Input: part model. Units: mm. Frame: model coordinates. Face numbers are marked on the shaded views. A direction names the side the tool comes from. Round coordinates to 2 decimals unless told otherwise and drop trailing zeros. Order: outer loops, then holes, each group sorted by start corner. A loop starts at its lowest first (then second) coordinate and runs counter-clockwise, first axis right, second up.
Item 1: First-contact query: pin 1 (3 mm diameter, centred on x = 9, y = -1, fed in from +Z); pin 2 (2 mm diameter, centred on y = -5, z = 5.5, fed in from +X); pin 3 (4.5 mm diameter, centred on x = 11, z = 3.5, fed in from -Y); pin 4 (1.6 mm diameter, centred on x = 10, y = -6, fed in from -Z). Flat tips, straight axial feed; report the tip coordinate or a pass-through.
Item 2: Mould query, pull axis Y, two halves, no side actions, for the marked faces 5, 6, 7 and 8. Classes: released by +Y, released by -Y, zero draft, split by the parting line, or undercut.
Item 3: Cut plane B-B on y = 7. Output: boundary loops of the cut face in (x, z).
Item 4: Line query: L1, parallel to Z at x = 4.75, y = -7.5; L2, parallel to Y at x = 5, z = 6 (3 decimals); L3, parallel to Y at x = -7.5, z = 3.6. Output: solid intervals per line, ascending.
Item 5: Cut plane C-C on x = 7.25. Output: boundary loops of the cut face in (y, z), then the cut area to 3 significant figures.
Item 6: Reachability of the marked faces 1, 2, 3 and 4 from +Z, -Z, +X, -X, +Y, -Y: full face, straight path, thin tool, end or side. Return the list, or none.
Item 7: Cut plane D-D on z = 2.75. Give the number of separate pieces and of enclosed holes in the cut face, then the cut area to 3 significant figures.
Item 8: Cut plane A-A on x = -9. Output: boundary loops of the cut face in (y, z).
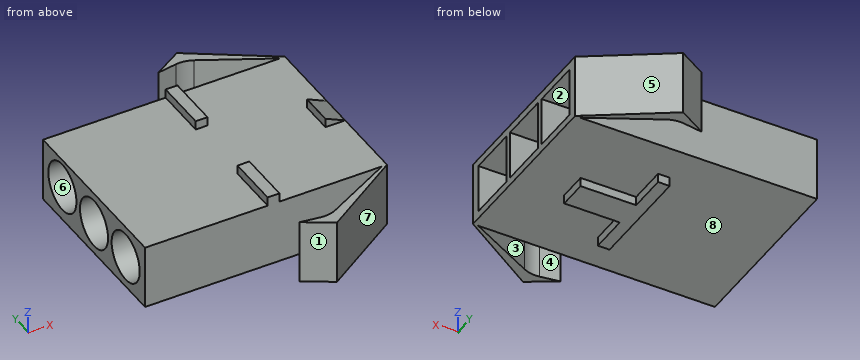
```python
from build123d import *

# Parameters (mm, degrees)
SKETCH_1_W          = 27
SKETCH_1_H          = 20
EXTRUDE_1_DEPTH     = 7.2
SKETCH_2_W          = 5.5
SKETCH_2_H          = 5.5
CUT_EXTRUDE_1_DEPTH = 10.2
SKETCH_3_R          = 2.75
CUT_EXTRUDE_2_DEPTH = 18
SKETCH_4_W          = 1.32
SKETCH_4_H          = 5.9
SKETCH_4_W_2        = 2.2
SKETCH_4_H_2        = 3.6
EXTRUDE_2_DEPTH     = 1
CHAMFER_1_SIZE      = 1
CHAMFER_1_SIZE2     = 2.144506921
EXTRUDE_4_DEPTH     = 1
EXTRUDE_5_DEPTH     = 7.2
FILLET_1_R          = 3
FILLET_2_R          = 3


with BuildPart() as part:
    # 草图1 → 凸台-拉伸1 (new body)
    with BuildSketch(Plane.XY):
        Rectangle(SKETCH_1_W, SKETCH_1_H)
    extrude(amount=EXTRUDE_1_DEPTH)

    # 草图2 → 切除-拉伸1 (cut)
    with BuildSketch(Plane(origin=(13.5, 0, 0), x_dir=(0, 0, -1), z_dir=(1, 0, 0))):
        with Locations((-3.6, -6.2)):
            Rectangle(SKETCH_2_W, SKETCH_2_H)
        with Locations((-3.6, 0)):
            Rectangle(SKETCH_2_W, SKETCH_2_H)
        with Locations((-3.6, 6.2)):
            Rectangle(SKETCH_2_W, SKETCH_2_H)
    extrude(amount=-CUT_EXTRUDE_1_DEPTH, mode=Mode.SUBTRACT)

    # 草图3 → 切除-拉伸2 (cut)
    with BuildSketch(Plane.ZY.offset(13.5)):
        with Locations((3.6, 0)):
            Circle(SKETCH_3_R)
        with Locations((3.920071901, 6.2)):
            Circle(SKETCH_3_R)
        with Locations((3.6, -6.2)):
            Circle(SKETCH_3_R)
    extrude(amount=-CUT_EXTRUDE_2_DEPTH, mode=Mode.SUBTRACT)

    # 草图4 → 凸台-拉伸2 (add)
    with BuildSketch(Plane.XY.offset(7.2)):
        with Locations((0.84, 7.05)):
            Rectangle(SKETCH_4_W, SKETCH_4_H)
        with Locations((0.84, -7.05)):
            Rectangle(SKETCH_4_W, SKETCH_4_H)
        with Locations((12.4, 0)):
            Rectangle(SKETCH_4_W_2, SKETCH_4_H_2)
    extrude(amount=EXTRUDE_2_DEPTH)

    # 倒角1
    chamfer_1_edges = [part.edges().sort_by_distance(p)[0] for p in [
        (13.5, 0, 8.2),
    ]]
    chamfer_1_side = [part.faces().sort_by_distance(p)[0] for p in [
        (13.5, -9.78384265, 3.6),
    ]]
    chamfer(chamfer_1_edges, length=CHAMFER_1_SIZE, length2=CHAMFER_1_SIZE2, reference=chamfer_1_side[0])

    # 草图6 → 凸台-拉伸4 (add)
    with BuildSketch(Plane(origin=(0, 0, 0), x_dir=(-1, 0, 0), z_dir=(0, 0, -1))):
        Polygon((-8.1, -1.6), (-8.1, 1.6), (-1.9, 1.6), (-1.9, 5.9), (-0.6, 5.9), (-0.6, -5.9), (-1.9, -5.9), (-1.9, -1.6), align=None)
    extrude(amount=EXTRUDE_4_DEPTH)

    # 草图7 → 凸台-拉伸5 (add)
    with BuildSketch(Plane(origin=(0, 0, 0), x_dir=(-1, 0, 0), z_dir=(0, 0, -1))):
        Polygon((-13.5, 10), (-4.675788996, 15.698556705), (-1.558596332, 13.847723561), (-4.675788996, 14.319689506), (-12.931993779, 10), align=None)
        Polygon((-12.931993779, -10), (-13.5, -10), (-4.675788996, -15.698556705), (-1.558596332, -13.847723561), (-4.675788996, -14.319689506), align=None)
    extrude(amount=-EXTRUDE_5_DEPTH)

    # 圆角1
    fillet_1_edges = [part.edges().sort_by_distance(p)[0] for p in [
        (4.675788996, 14.319689506, 3.6),
    ]]
    fillet(fillet_1_edges, radius=FILLET_1_R)

    # 圆角2
    fillet_2_edges = [part.edges().sort_by_distance(p)[0] for p in [
        (4.675788996, -14.319689506, 3.6),
    ]]
    fillet(fillet_2_edges, radius=FILLET_2_R)


solid = part.part
```
From the geometry:
1. pin 1: stops at z = 7.2
1. pin 2: stops at x = 13.5
1. pin 3: stops at y = -13.07
1. pin 4: stops at z = 0
2. face 5: released by +Y
2. face 6: undercut
2. face 7: released by -Y
2. face 8: zero draft
3. outline: (-13.5, 0) - (13.5, 0) - (13.5, 0.85) - (3.3, 0.85) - (3.3, 1.29) - (-13.5, 1.29) - close; (-13.5, 6.55) - (4.5, 6.55) - (4.5, 6.35) - (13.5, 6.35) - (13.5, 7.2) - (1.5, 7.2) - (1.5, 8.2) - (0.18, 8.2) - (0.18, 7.2) - (-13.5, 7.2) - close
4. L1: z = 0 to 0.85, 6.35 to 7.2
4. L2: y = -15.489 to -14.085, -10 to -8.95, -3.45 to -2.75, 2.75 to 3.45, 8.95 to 10, 14.085 to 15.489
4. L3: y = -10 to -8.95, -3.45 to -2.75, 2.75 to 3.47, 8.93 to 10
5. outline: (-14.04, 0) - (-12.97, 0) - (-12.97, 7.2) - (-14.04, 7.2) - close; (-10, 0) - (-1.6, 0) - (-1.6, -1) - (1.6, -1) - (1.6, 0) - (10, 0) - (10, 7.2) - (-10, 7.2) - close; (12.97, 0) - (14.04, 0) - (14.04, 7.2) - (12.97, 7.2) - close; hole (-8.95, 0.85) - (-3.45, 0.85) - (-3.45, 6.35) - (-8.95, 6.35) - close; hole (-2.75, 0.85) - (2.75, 0.85) - (2.75, 6.35) - (-2.75, 6.35) - close; hole (3.45, 0.85) - (8.95, 0.85) - (8.95, 6.35) - (3.45, 6.35) - close
5. area: 71.8 mm2
6. face 1: +Z, -Z, -X, -Y
6. face 2: +X
6. face 3: +Z, -Z, -X
6. face 4: +Z, -Z
7. separate pieces: 4
7. enclosed holes: 0
7. area: 131 mm2
8. outline: (-10, 0) - (10, 0) - (10, 7.2) - (-10, 7.2) - close; hole circle Ø5.5 at (-6.2, 3.6); hole circle Ø5.5 at (0, 3.6); hole circle Ø5.5 at (6.2, 3.92)
